Geometry: final body of the model. Coordinates: model frame, mm. Face numbers are marked on the shaded views. A direction names the side the tool comes from. Round coordinates to 2 decimals unless told otherwise and drop trailing zeros. Loops run counter-clockwise (first coordinate to the right, second up) from the corner with the lowest first, then second, coordinate; pieces in that order, holes last. Notation, with made-up numbers: (54.5, -27) - (66.5, -27) arc R31 cw to (66.5, -1) - close; hole circle Ø3 at (-37, -9). An arc over 180 degrees is marked (long way). Answer in a Markdown table with one row per item. Add a question column.
from build123d import *

# Parameters (mm, degrees)
BOSS_EXTRUDE2_DEPTH = 50.8
CUT_EXTRUDE1_REACH  = 68.632
SKETCH3_R           = 4.7625
SKETCH4_R           = 4.7625
BOSS_EXTRUDE3_DEPTH = 12.7


with BuildPart() as part:
    # Sketch2 → Boss-Extrude2 (new body)
    with BuildSketch(Plane(origin=(0, 0, 0), x_dir=(0, 0, -1), z_dir=(1, 0, 0))):
        Polygon((-25.4, 0), (25.4, 0), (46.869007696, 46.040435581), (41.113953249, 48.724061544), (21.354603844, 6.35), (-25.4, 6.35), align=None)
    extrude(amount=BOSS_EXTRUDE2_DEPTH)

    # Sketch3 → Cut-Extrude1 (cut, up to next)
    with BuildSketch(Plane(origin=(0, -9.728764428, -20.863402643), x_dir=(1, 0, 0), z_dir=(0, -0.422618262, -0.906307787)), mode=Mode.PRIVATE) as cut_extrude1_sk1:
        with Locations((25.4, -48.834503848)):
            Circle(SKETCH3_R)
    cut_extrude1_tool1 = extrude(cut_extrude1_sk1.sketch, amount=-CUT_EXTRUDE1_REACH, mode=Mode.PRIVATE) & part.part
    add(cut_extrude1_tool1.solids().sort_by_distance((25.4, 34.530327, -41.501756))[0], mode=Mode.SUBTRACT)

    # Sketch4 → Boss-Extrude3 (add)
    with BuildSketch(Plane.XZ):
        with Locations((25.4, 0)):
            Circle(SKETCH4_R)
    extrude(amount=BOSS_EXTRUDE3_DEPTH)


solid = part.part
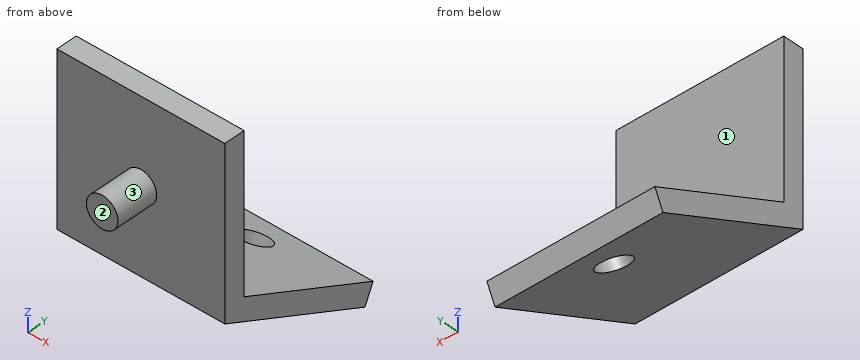
1) Section A-A, the plane x = 28.5. Return the cut outline in (y, z), and give its area (3 significant figures).
2) Section B-B, the plane z = 0. Return the cut outline in (x, y), and give its area (3 significant figures).
3) Reachability of the marked faces 1, 2 and 3 from +Z, -Z, +X, -X, +Y, -Y: full face, straight path, thin tool, end or side. Return the list, or none.
4) Section C-C, the plane x = 18.5. Return the cut outline in (y, z), and give its area (3 significant figures).
5) Material intervals for line 1 along Y through (x, z) = (29, -2.5); line 2 along Y through (x, z) = (7, 14); line 3 along Z through (x, y) = (34.5, 39), sorted ascending. Write a range as from..to.
6) Section D-D, the plane y = 4. Return the cut outline in (x, z), and give its area (3 significant figures).
7) Contact query for flat-ended pins moving along their axis: pin 1 Ø5 at (x, z) = (14.5, 3) entering from +Y; pin 2 Ø1 at (x, y) = (8, 41) entering from +Z; pin 3 Ø4 at (x, y) = (15.5, 42.5) entering from -Z. Output: stop coordinate, or through.
Evaluation:
| question | item | result |
|---|---|---|
| 1 | outline | (-12.7, -3.62) - (0, -3.62) - (0, -25.4) - (31.25, -39.97) - (33.94, -34.22) - (6.35, -21.35) - (6.35, 25.4) - (0, 25.4) - (0, 3.62) - (-12.7, 3.62) - close; (37.81, -43.03) - (46.04, -46.87) - (48.72, -41.11) - (40.49, -37.27) - close |
| 1 | area | 665 mm² |
| 2 | outline | (0, 0) - (20.64, 0) - (20.64, -12.7) - (30.16, -12.7) - (30.16, 0) - (50.8, 0) - (50.8, 6.35) - (0, 6.35) - close |
| 2 | area | 444 mm² |
| 3 | face 1 | +Z, +X, -X, +Y |
| 3 | face 2 | +Z, -Z, +X, -X, -Y |
| 3 | face 3 | -Y |
| 4 | outline | (0, -25.4) - (46.04, -46.87) - (48.72, -41.11) - (6.35, -21.35) - (6.35, 25.4) - (0, 25.4) - close |
| 4 | area | 619 mm² |
| 5 | line 1 | y = -12.7..6.35 |
| 5 | line 2 | y = 0..6.35 |
| 5 | line 3 | z = -43.59..-36.58 |
| 6 | outline | (0, -27.27) - (50.8, -27.27) - (50.8, 25.4) - (0, 25.4) - close |
| 6 | area | 2,680 mm² |
| 7 | pin 1 | stops at y = 6.35 |
| 7 | pin 2 | stops at z = -37.28 |
| 7 | pin 3 | stops at z = -46.15 |
